```python
from build123d import *

# Parameters (mm, degrees)
SKETCH1_R           = 42.075
BOSS_EXTRUDE1_DEPTH = 15
BOSS_EXTRUDE3_DEPTH = 20
SKETCH10_R          = 4
BOSS_EXTRUDE8_DEPTH = 8


with BuildPart() as part:
    # Sketch1 → Boss-Extrude1 (new body)
    with BuildSketch(Plane.XY):
        Circle(SKETCH1_R)
    extrude(amount=BOSS_EXTRUDE1_DEPTH)

    # Sketch4 → Boss-Extrude3 (add)
    with BuildSketch(Plane(origin=(0, 0, 0), x_dir=(-1, 0, 0), z_dir=(0, 0, -1))):
        Polygon((10, 0), (0, 0), (-15, 0), (-15, -60), (10, -60), align=None)
    extrude(amount=BOSS_EXTRUDE3_DEPTH)

    # Sketch10 → Boss-Extrude8 (add)
    with BuildSketch(Plane(origin=(0, 0, -20), x_dir=(-1, 0, 0), z_dir=(0, 0, -1))):
        with Locations((-3.69323872, -55.331161555)):
            Circle(SKETCH10_R)
    extrude(amount=BOSS_EXTRUDE8_DEPTH)


solid = part.part
```
Could you check a few things on this model? Use its own coordinates, in mm. A direction names the side the tool comes from. Round coordinates to 2 decimals unless told otherwise and drop trailing zeros. Loops run counter-clockwise (first coordinate to the right, second up) from the corner with the lowest first, then second, coordinate; pieces in that order, holes last.
Q1. I want a section at D-D (y = -50). Write out the boundary of the cut face in (x, z), and give its area (3 significant figures).
Q2. I want a section at A-A (y = -19). Write out the boundary of the cut face in (x, z), and give its area (3 significant figures).
Q3. I want a section at C-C (z = -22). Write out the boundary of the cut face in (x, y).
Q4. Please list where these lines run through material, in increasing order: L1, parallel to Y at x = 11, z = -4.5; L2, parallel to Z at x = 2, y = 4.5; L3, parallel to X at y = -8.5, z = -3.5.
Q5. Thinking about a two-plate mould opening in Y: for faces 1 (the flat face through (2, 0, -10)), 2 (the cylindrical face through (-5.477, 41.717, 7.395)), 3 (the flat face through (4, -55, -28)), which applies, pulls with the +Y half, pulls with the -Y half, needs draft (parallel to the pull), parting line crosses it, or undercut?
Q6. On a 3-axis mill with a long thin cutter (end or side, diameter ignored), from which of +Z, -Z, +X, -X, +Y, -Y can I reach the whole of each face in a straight line? I mean faces 4 (the flat face through (15, -30, -10)), 5 (the flat face through (-10, -30, -10)), 6 (the cylindrical face through (4.214, -51.365, -23.944)), 7 (the flat face through (-1, 1, 15)). Say none if no direction works.
Q7. For P1, Ø16, axis at x = 4, z = -14.5, coming from the +Y side; P2, Ø12, axis at x = -7.5, y = 20.5, coming from the -Z side; P3, Ø10, axis at y = -22.5, z = -11, coming from the -X side, each with a flat end and sliding along its axis, tell me the tip position at first contact or that it passes through.
Q8. I want a section at B-B (x = -2.5). Write out the boundary of the cut face in (y, z).
Answer below:
1. outline: (-10, -20) - (15, -20) - (15, 0) - (-10, 0) - close
1. area: 500 mm2
2. outline: (-37.54, 0) - (-10, 0) - (-10, -20) - (15, -20) - (15, 0) - (37.54, 0) - (37.54, 15) - (-37.54, 15) - close
2. area: 1,630 mm2
3. outline: circle Ø8 at (3.69, -55.33)
4. L1: y = -60 to 0
4. L2: z = 0 to 15
4. L3: x = -10 to 15
5. face 1: pulls with the +Y half
5. face 2: parting line crosses it
5. face 3: needs draft
6. face 4: -Z, +X, +Y, -Y
6. face 5: -Z, -X, +Y, -Y
6. face 6: -Z
6. face 7: +Z, +X, -X, +Y, -Y
7. P1: stops at y = 0
7. P2: stops at z = 0
7. P3: stops at x = -10
8. outline: (-60, -20) - (0, -20) - (0, 0) - (42, 0) - (42, 15) - (-42, 15) - (-42, 0) - (-60, 0) - close
